Build history of the part. All positions in model axes, mm. Round coordinates to 2 decimals unless told otherwise and drop trailing zeros. Order: outer loops, then holes, each group sorted by start corner. A loop starts at its lowest first (then second) coordinate and runs counter-clockwise, first axis right, second up. Notation, with made-up numbers: (50, 10.5) -> (70, 10.5) arc R29 cw to (70, 35.5) -> close; hole circle Ø5 at (75.25, 76.25). An arc over 180 degrees is marked (long way). Use a Markdown table: item, result. Add a question column.
Item 1: Slice it at D-D, the plane x = -15.5. Give the cut face in (y, z), plus the area to 3 significant figures.
Item 2: Slice it at C-C, the plane y = 19.05. Give the cut face in (x, z), plus the area to 3 significant figures.
Item 3: Two-plate mould, pull along Y, no slides. Class faces 1 (the face through (3.03, 0.95, 1.22)), 2 (the face through (-5.506, -24.796, 2.504)), 3 (the face through (1.292, -3.116, 2.583)), 4 (the face through (5, 0, 0)): released by +Y, released by -Y, zero draft, split by the parting line, or undercut.
Item 4: Probe L1, parallel to Y at x = 0, z = 1.35 (3 decimals); L2, parallel to Y at x = -0.5, z = 2.5; L3, parallel to X at y = 19.5, z = 4.3. List the from-to ranges inside material, lowest first.
Item 5: Slice it at B-B, the plane x = 0. Give the cut face in (y, z) (3 decimals).
Item 6: Slice it at A-A, the plane y = 0. Give the cut face in (x, z) (3 decimals).
from build123d import *

# Parameters (mm, degrees)
SKETCH1_R             = 25.4
DISC_BASE_DEPTH       = 5.08
SKETCH2_R             = 3.175
CUT_EXTRUDE2_DEPTH    = 37.278456417
F_6_32_TAPPED_HOLE1_D = 2.7051


with BuildPart() as part:
    # Sketch1 → Disc Base (new body)
    with BuildSketch(Plane.XY):
        Circle(SKETCH1_R)
    extrude(amount=DISC_BASE_DEPTH)

    # Sketch10 → CSK for 1/4 Flat Head Machine Screw (100)1 (revolve, cut)
    with BuildSketch(Plane(origin=(0, 0, 5.08), x_dir=(0, -1, 0), z_dir=(1, 0, 0))):
        Polygon((0, 0), (0, 2.54), (3.175, 0.632267535), (3.175, 2.664141329), (6.35, 0), align=None)
    revolve(axis=Axis((0, 0, 11.43), (0, 0, -1)), mode=Mode.SUBTRACT)

    # Sketch2 → Cut-Extrude2 (cut, through all)
    with BuildSketch(Plane.XY.offset(5.08)):
        Circle(SKETCH2_R)
    extrude(amount=-CUT_EXTRUDE2_DEPTH, mode=Mode.SUBTRACT)

    # #6-32 Tapped Hole1 (through all)
    with Locations(Plane(origin=(0, 19.05, 5.08), x_dir=(1, 0, 0), z_dir=(0, 0, 1))):
        with Locations((0, 0)):
            Hole(F_6_32_TAPPED_HOLE1_D / 2)


solid = part.part
Check sheet entries:
| question | item | result |
|---|---|---|
| 1 | outline | (-20.12, 0) -> (20.12, 0) -> (20.12, 5.08) -> (-20.12, 5.08) -> close |
| 1 | area | 204 mm2 |
| 2 | outline | (-16.8, 0) -> (-1.35, 0) -> (-1.35, 5.08) -> (-16.8, 5.08) -> close; (1.35, 0) -> (16.8, 0) -> (16.8, 5.08) -> (1.35, 5.08) -> close |
| 2 | area | 157 mm2 |
| 3 | face 1 | undercut |
| 3 | face 2 | split by the parting line |
| 3 | face 3 | undercut |
| 3 | face 4 | zero draft |
| 4 | L1 | -25.4 to -3.175, 3.175 to 17.697, 20.403 to 25.4 |
| 4 | L2 | -25.4 to -3.24, 3.24 to 17.79, 20.31 to 25.4 |
| 4 | L3 | -16.28 to -1.28, 1.28 to 16.28 |
| 5 | outline | (-25.4, 0) -> (-3.175, 0) -> (-3.175, 2.416) -> (-6.35, 5.08) -> (-25.4, 5.08) -> close; (3.175, 0) -> (17.697, 0) -> (17.697, 5.08) -> (6.35, 5.08) -> (3.175, 2.416) -> close; (20.403, 0) -> (25.4, 0) -> (25.4, 5.08) -> (20.403, 5.08) -> close |
| 6 | outline | (-25.4, 0) -> (-3.175, 0) -> (-3.175, 2.416) -> (-6.35, 5.08) -> (-25.4, 5.08) -> close; (3.175, 0) -> (25.4, 0) -> (25.4, 5.08) -> (6.35, 5.08) -> (3.175, 2.416) -> close |
